```python
from build123d import *

# Parameters (mm, degrees)
SKIZZE1_R                       = 5
SKIZZE1_R_2                     = 2.75
SKIZZE1_W                       = 43.1
SKIZZE1_H                       = 63
AUFSATZ_LINEAR_AUSTRAGEN1_DEPTH = 10
SKIZZE3_W                       = 200
SKIZZE3_H                       = 15
AUFSATZ_LINEAR_AUSTRAGEN2_DEPTH = 150
VERRUNDUNG1_R                   = 10
AUFSATZ_LINEAR_AUSTRAGEN3_DEPTH = 10
AUFSATZ_LINEAR_AUSTRAGEN4_DEPTH = 10


with BuildPart() as part:
    # Skizze1 → Aufsatz-Linear austragen1 (new body)
    with BuildSketch(Plane(origin=(0, 0, 0), x_dir=(1, 0, 0), z_dir=(0, 1, 0))):
        with BuildLine():
            Line((-125, 100), (125, 100))
            ThreePointArc((125, 100), (132.071067812, 97.071067812), (135, 90))
            Line((135, 90), (135, 60))
            ThreePointArc((135, 60), (132.071067812, 52.928932188), (125, 50))
            Line((125, 50), (80, 50))
            ThreePointArc((80, 50), (69.393398282, 45.606601718), (65, 35))
            Line((65, 35), (65, -70))
            ThreePointArc((65, -70), (69.393398282, -80.606601718), (80, -85))
            Line((80, -85), (90, -85))
            Line((90, -85), (100, -85))
            Line((100, -85), (100, -100))
            Line((100, -100), (80, -100))
            Line((80, -100), (-80, -100))
            Line((-80, -100), (-100, -100))
            Line((-100, -100), (-100, -85))
            Line((-100, -85), (-90, -85))
            Line((-90, -85), (-80, -85))
            ThreePointArc((-80, -85), (-69.393398282, -80.606601718), (-65, -70))
            Line((-65, -70), (-65, 35))
            ThreePointArc((-65, 35), (-69.393398282, 45.606601718), (-80, 50))
            Line((-80, 50), (-125, 50))
            ThreePointArc((-125, 50), (-132.071067812, 52.928932188), (-135, 60))
            Line((-135, 60), (-135, 90))
            ThreePointArc((-135, 90), (-132.071067812, 97.071067812), (-125, 100))
        make_face()
        with Locations(Location((-105, 75, 0), (0, 0, 270))):
            Circle(SKIZZE1_R, mode=Mode.SUBTRACT)
        with Locations(Location((105, 75, 0), (0, 0, 90))):
            Circle(SKIZZE1_R, mode=Mode.SUBTRACT)
        with Locations(Location((-97.5, 82.5, 0), (0, 0, 270))):
            Circle(SKIZZE1_R_2, mode=Mode.SUBTRACT)
        with Locations(Location((-112.5, 67.5, 0), (0, 0, 270))):
            Circle(SKIZZE1_R_2, mode=Mode.SUBTRACT)
        with Locations(Location((97.5, 82.5, 0), (0, 0, 90))):
            Circle(SKIZZE1_R_2, mode=Mode.SUBTRACT)
        with Locations(Location((112.5, 67.5, 0), (0, 0, 90))):
            Circle(SKIZZE1_R_2, mode=Mode.SUBTRACT)
        with Locations((0, 42.21)):
            Rectangle(SKIZZE1_W, SKIZZE1_H, mode=Mode.SUBTRACT)
    extrude(amount=AUFSATZ_LINEAR_AUSTRAGEN1_DEPTH)

    # Skizze3 → Aufsatz-Linear austragen2 (add)
    with BuildSketch(Plane(origin=(0, 10, 0), x_dir=(1, 0, 0), z_dir=(0, 1, 0))):
        with Locations((0, -92.5)):
            Rectangle(SKIZZE3_W, SKIZZE3_H)
    extrude(amount=AUFSATZ_LINEAR_AUSTRAGEN2_DEPTH)

    # Verrundung1
    verrundung1_edges = [part.edges().sort_by_distance(p)[0] for p in [
        (-100, 160, 92.5),
        (100, 160, 92.5),
        (100, 0, 92.5),
        (-100, 0, 92.5),
    ]]
    fillet(verrundung1_edges, radius=VERRUNDUNG1_R)

    # Skizze5 → Aufsatz-Linear austragen3 (add)
    with BuildSketch(Plane.ZY.offset(50)):
        Polygon((15, 10), (85, 80), (85, 10), align=None)
    extrude(amount=-AUFSATZ_LINEAR_AUSTRAGEN3_DEPTH)

    # Skizze6 → Aufsatz-Linear austragen4 (add)
    with BuildSketch(Plane(origin=(55, 0, 0), x_dir=(0, 0, -1), z_dir=(1, 0, 0))):
        Polygon((-15, 10), (-85, 80), (-85, 10), align=None)
    extrude(amount=-AUFSATZ_LINEAR_AUSTRAGEN4_DEPTH)


solid = part.part
```
Could you check a few things on this model? Use its own coordinates, in mm. A direction names the side the tool comes from. Round coordinates to 2 decimals unless told otherwise and drop trailing zeros. Loops run counter-clockwise (first coordinate to the right, second up) from the corner with the lowest first, then second, coordinate; pieces in that order, holes last. Notation, with made-up numbers: (15.25, 36) - (37.25, 36) arc R26 ccw to (37.25, 53) - close; hole circle Ø3 at (9.25, 37). An arc over 180 degrees is marked (long way). Answer in a Markdown table with one row per item. Add a question column.
(1) I need wall thicknesses on line 1 along X through (y, z) = (6, -75); line 2 along X through (y, z) = (2, -82.5); line 3 along Y through (x, z) = (48, -76). Which ranges of each line are inside material? Lowest first, please.
(2) I'm going to push flat-ended pins straight in: pin 1 (6.5 mm diameter, centred on x = 112.5, z = -67.5, fed in from +Y); pin 2 (7.5 mm diameter, centred on y = 64.5, z = 91, fed in from +X); pin 3 (5 mm diameter, centred on y = 5.5, z = -46, fed in from -X). Where does each tip first touch, or does it pass through?
(3) If we section it at B-B (z = -19): Please give me the cut outline in (x, y), plus the area to 3 significant figures.
(4) If we section it at C-C (y = 50.5): Please give me the cut outline in (x, z).
(5) If we section it at A-A (x = -13): Please give me the cut outline in (y, z), plus the area to 3 significant figures.
(6) If we mould it in two halves opening along Z, with no side actions, what happens to faces 5 (the face through (-21.55, 5, -42)), 6 (the face through (50, 45, 50)), 7 (the face through (-102, 5, -50)), 8 (the face through (2, 10, -9))? For each: pulls with the +Z half, pulls with the -Z half, needs draft (parallel to the pull), parting line crosses it, or undercut.
(7) For faces 1 (the face through (69.51, 4.93, -45.72)), 2 (the face through (97.15, 156.99, 92.4)), 3 (the face through (-65, 5, 18)), 4 (the face through (0, 5, -73.71)), which set-ups out of +Z, -Z, +X, -X, +Y, -Y let a thin tool reach every point of the face, with its end or its side?
(8) If we section it at D-D (z = 29): Please give me the cut outline in (x, y).
Model answer:
| question | item | result |
|---|---|---|
| 1 | line 1 | x = -135 to -110, -100 to 100, 110 to 135 |
| 1 | line 2 | x = -135 to -100.25, -94.75 to 94.75, 100.25 to 135 |
| 1 | line 3 | y = 0 to 10 |
| 2 | pin 1 | stops at y = 10 |
| 2 | pin 2 | stops at x = 100 |
| 2 | pin 3 | stops at x = -73.46 |
| 3 | outline | (-65, 0) - (-21.55, 0) - (-21.55, 10) - (-65, 10) - close; (21.55, 0) - (65, 0) - (65, 10) - (21.55, 10) - close |
| 3 | area | 869 mm² |
| 4 | outline | (-100, 85) - (-50, 85) - (-50, 55.5) - (-40, 55.5) - (-40, 85) - (45, 85) - (45, 55.5) - (55, 55.5) - (55, 85) - (100, 85) - (100, 100) - (-100, 100) - close |
| 5 | outline | (0, -100) - (10, -100) - (10, -73.71) - (0, -73.71) - close; (0, -10.71) - (10, -10.71) - (10, 85) - (160, 85) - (160, 100) - (0, 100) - close |
| 5 | area | 3,620 mm² |
| 6 | face 5 | undercut |
| 6 | face 6 | pulls with the -Z half |
| 6 | face 7 | undercut |
| 6 | face 8 | needs draft |
| 7 | face 1 | +X, +Y, -Y |
| 7 | face 2 | +Z, -Z, +X, +Y |
| 7 | face 3 | -X, +Y, -Y |
| 7 | face 4 | +Y, -Y |
| 8 | outline | (-65, 0) - (65, 0) - (65, 10) - (55, 10) - (55, 24) - (45, 24) - (45, 10) - (-40, 10) - (-40, 24) - (-50, 24) - (-50, 10) - (-65, 10) - close |
